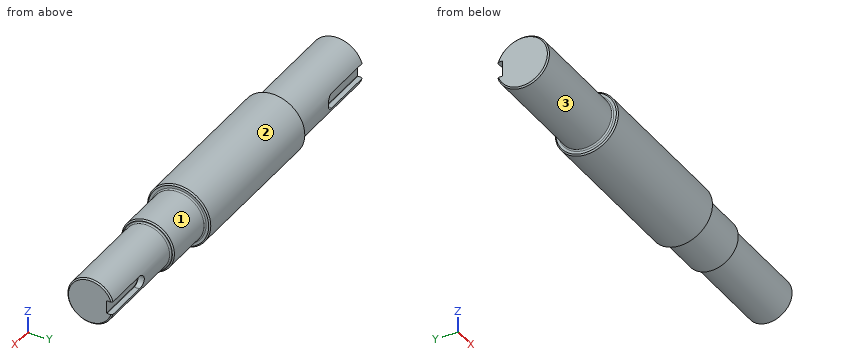
from build123d import *

# Parameters (mm, degrees)
CUT_EXTRUDE1_DEPTH = 5
FILLET1_R          = 0.3
CUT_EXTRUDE2_DEPTH = 5
FILLET2_R          = 0.3
CHAMFER1_SIZE      = 1
FILLET3_R          = 1


with BuildPart() as part:
    # Sketch1 → Revolve1 (revolve)
    with BuildSketch(Plane.XY):
        Polygon((-150, 0), (-150, 20), (-68, 20), (-68, 24), (55, 24), (55, 20), (95, 20), (95, 17.5), (168.5, 17.5), (168.5, 0), (34, 0), align=None)
    revolve(axis=Axis((-150, 0, 0), (1, 0, 0)))

    # Sketch2 → Cut-Extrude1 (cut)
    with BuildSketch(Plane(origin=(0, 20, 0), x_dir=(1, 0, 0), z_dir=(0, 1, 0))):
        with BuildLine():
            Line((-150, 6), (-150, -6))
            Line((-150, -6), (-110, -6))
            ThreePointArc((-110, -6), (-104, 0), (-110, 6))
            Line((-110, 6), (-150, 6))
        make_face()
    extrude(amount=-CUT_EXTRUDE1_DEPTH, mode=Mode.SUBTRACT)

    # Fillet1
    fillet1_edges = [part.edges().sort_by_distance(p)[0] for p in [
        (-130, 15, 6),
        (-104, 15, 0),
        (-130, 15, -6),
    ]]
    fillet(fillet1_edges, radius=FILLET1_R)

    # Sketch3 → Cut-Extrude2 (cut)
    with BuildSketch(Plane(origin=(0, 17.5, 0), x_dir=(1, 0, 0), z_dir=(0, 1, 0))):
        with BuildLine():
            Line((168.5, -5), (168.5, 5))
            Line((168.5, 5), (133.5, 5))
            ThreePointArc((133.5, 5), (128.5, 0), (133.5, -5))
            Line((133.5, -5), (168.5, -5))
        make_face()
    extrude(amount=-CUT_EXTRUDE2_DEPTH, mode=Mode.SUBTRACT)

    # Fillet2
    fillet2_edges = [part.edges().sort_by_distance(p)[0] for p in [
        (128.5, 12.5, 0),
        (151, 12.5, -5),
        (151, 12.5, 5),
    ]]
    fillet(fillet2_edges, radius=FILLET2_R)

    # Chamfer1
    chamfer1_edges = [part.edges().sort_by_distance(p)[0] for p in [
        (95, -20, 0),
        (55, -24, 0),
        (-68, -24, 0),
        (-150, -20, 0),
        (168.5, -17.5, 0),
    ]]
    chamfer(chamfer1_edges, length=CHAMFER1_SIZE)

    # Fillet3
    fillet3_edges = [part.edges().sort_by_distance(p)[0] for p in [
        (55, -20, 0),
        (-68, -20, 0),
        (95, -17.5, 0),
    ]]
    fillet(fillet3_edges, radius=FILLET3_R)


solid = part.part
The model under review builds one solid part; all positions refer to its coordinate system, in mm. Face numbers are marked on the shaded views. A direction names the side the tool comes from. Coordinates: 2 decimals unless noted, no trailing zeros. Write each loop counter-clockwise with the first axis right and the second up, starting at its lowest first coordinate (ties: lowest second). Pieces come first, ordered by that corner, then holes. Notation, with made-up numbers: (78, 49) - (84, 49) arc R16 cw to (84, 73) - close; hole circle Ø6 at (4, -38.75). An arc over 180 degrees is marked (long way). Answer as a JSON object with one key per item and string values. Group by question number.
1. Add section B-B (x = -119.5). Give the boundary of the cut face in (y, z), plus the area to 3 significant figures.
2. Machinability: for the marked faces 1, 2 and 3, which of the approach directions +Z, -Z, +X, -X, +Y, -Y give a long, thin tool a straight path to every point of the face, cutting with its end or side? Answer none if there is none.
3. Add section D-D (x = 148). Give the boundary of the cut face in (y, z).
4. Add section C-C (x = -56.5). Give the boundary of the cut face in (y, z).
5. Clearance check with flat-ended pins moving along their axes: pin 1 Ø1 at (y, z) = (14.5, 18) entering from +X; pin 2 Ø4.5 at (x, y) = (159, 15.5) entering from -Z; pin 3 Ø6 at (x, y) = (-91.5, 13.5) entering from +Z. State where each tip first meets the part, or that it passes through.
6. To check wall thickness, follow probe 1 along Y at (x, z) = (-92.5, 0.5); probe 2 along X at (y, z) = (7, -17); probe 3 along Y at (x, z) = (-90, 1.5). State the ranges of each line that lie inside material, in increasing order.
Findings:
{
 "1": {"outline": "(15, -5.7) - (15, 5.7) arc R0.3 cw to (15.3, 6) - (19.08, 6) arc R20 ccw (long way) to (19.08, -6) - (15.3, -6) arc R0.3 cw to start", "area": "1,200 mm²"},
 "2": {"face 1": "+X", "face 2": "+X, -X", "face 3": "-X"},
 "3": {"outline": "(12.5, -4.7) - (12.5, 4.7) arc R0.3 cw to (12.8, 5) - (16.77, 5) arc R17.5 ccw (long way) to (16.77, -5) - (12.8, -5) arc R0.3 cw to start"},
 "4": {"outline": "circle Ø48 at (0, 0)"},
 "5": {"pin 1": "x = 55", "pin 2": "z = -11.43", "pin 3": "z = 17.02"},
 "6": {"probe 1": "-19.99 to 19.99", "probe 2": "-150 to 95.01", "probe 3": "-19.94 to 19.94"}
}
